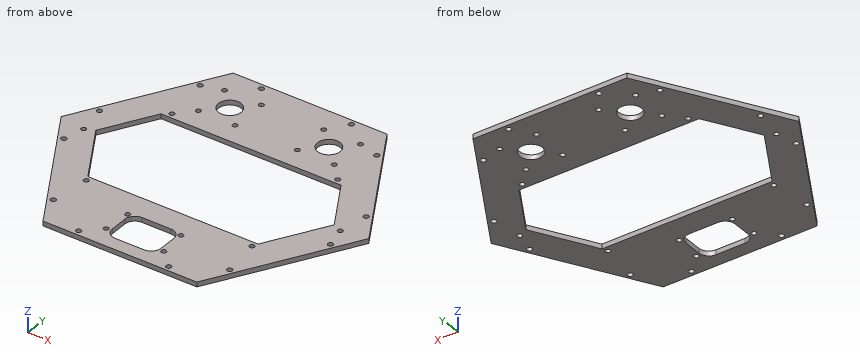
from build123d import *

# Parameters (mm, degrees)
FLANGE_BASE1_DEPTH          = 3.175
ESBO_O6_R                   = 1.65
CORTE_EXTRUS_O1_DEPTH       = 10
ESBO_O7_R                   = 1.75
CORTE_EXTRUS_O2_DEPTH       = 10
ESBO_O8_R                   = 7.554969153
ESBO_O8_R_2                 = 1.65
CORTE_EXTRUS_O3_DEPTH       = 10
PADR_OCIRCULAR1_COUNT       = 4
PADR_OCIRCULAR2_COUNT       = 6
ESPELHAR1_COPY_1_SKETCH_R   = 7.554969153
ESPELHAR1_COPY_1_SKETCH_R_2 = 1.65
ESPELHAR1_COPY_1_DEPTH      = 10
ESPELHAR1_COPY_2_SKETCH_R   = 7.554969153
ESPELHAR1_COPY_2_SKETCH_R_2 = 1.65
ESPELHAR1_COPY_2_DEPTH      = 10
ESPELHAR1_COPY_3_SKETCH_R   = 7.554969153
ESPELHAR1_COPY_3_SKETCH_R_2 = 1.65
ESPELHAR1_COPY_3_DEPTH      = 10
ESBO_O9_R                   = 1.65
CORTE_EXTRUS_O4_DEPTH       = 10


# Sheet-metal steps are written as plain solids
with BuildPart() as part:
    # Esboço1 → Flange-base1 (new body)
    with BuildSketch(Plane.XY):
        Polygon((51.251383396, 88.77), (102.502766792, 0), (51.251383396, -88.77), (-51.251383396, -88.77), (-102.502766792, 0), (-51.251383396, 88.77), align=None)
        Polygon((60, 33.616951546), (-60, 33.616951546), (-79.408756024, 0), (-56.734237399, -39.273418297), (56.734237399, -39.273418297), (79.408756024, 0), align=None, mode=Mode.SUBTRACT)
    extrude(amount=-FLANGE_BASE1_DEPTH)

    # Esboço6 → Corte-extrusão1 (cut)
    with BuildSketch(Plane.XY):
        with BuildLine():
            Line((9.692826752, -79.77), (-9.607173248, -79.77))
            ThreePointArc((-9.607173248, -79.77), (-14.274078004, -77.836904756), (-16.207173248, -73.17))
            Line((-16.207173248, -73.17), (-16.207173248, -61.37))
            ThreePointArc((-16.207173248, -61.37), (-14.274078004, -56.703095244), (-9.607173248, -54.77))
            Line((-9.607173248, -54.77), (9.692826752, -54.77))
            ThreePointArc((9.692826752, -54.77), (14.359731508, -56.703095244), (16.292826752, -61.37))
            Line((16.292826752, -61.37), (16.292826752, -73.17))
            ThreePointArc((16.292826752, -73.17), (14.359731508, -77.836904756), (9.692826752, -79.77))
        make_face()
        with Locations((-17.7, -56.67)):
            Circle(ESBO_O6_R)
        with Locations((17.7, -56.67)):
            Circle(ESBO_O6_R)
        with Locations((19.2, -74.77)):
            Circle(ESBO_O6_R)
        with Locations((-19.2, -74.77)):
            Circle(ESBO_O6_R)
    extrude(amount=-CORTE_EXTRUS_O1_DEPTH, mode=Mode.SUBTRACT)

    # Esboço7 → Corte-extrusão2 (cut)
    with BuildSketch(Plane.XY):
        with Locations((-30, -85.27)):
            Circle(ESBO_O7_R)
        with Locations((30, -85.27)):
            Circle(ESBO_O7_R)
    corte_extrus_o2 = extrude(amount=-CORTE_EXTRUS_O2_DEPTH, mode=Mode.SUBTRACT)

    # Esboço8 → Corte-extrusão3 (cut)
    with BuildSketch(Plane.XY):
        with Locations((-33, 60.0982)):
            Circle(ESBO_O8_R)
        with Locations((-20.75, 47.8482)):
            Circle(ESBO_O8_R_2)
    corte_extrus_o3 = extrude(amount=-CORTE_EXTRUS_O3_DEPTH, mode=Mode.SUBTRACT)

    # PadrãoCircular1: Corte-extrusão3 ×4 about axis
    padr_ocircular1_axis = Axis((-33, 60.0982, 0), (0, 0, 1))
    for i in range(1, PADR_OCIRCULAR1_COUNT):
        add(corte_extrus_o3.rotate(padr_ocircular1_axis, i * 360 / PADR_OCIRCULAR1_COUNT), mode=Mode.SUBTRACT)

    # PadrãoCircular2: Corte-extrusão2 ×6 about axis
    padr_ocircular2_axis = Axis((0, 0, 0), (0, 0, 1))
    for i in range(1, PADR_OCIRCULAR2_COUNT):
        add(corte_extrus_o2.rotate(padr_ocircular2_axis, i * 360 / PADR_OCIRCULAR2_COUNT), mode=Mode.SUBTRACT)

    # Espelhar1: Corte-extrusão3 across plane
    add(corte_extrus_o3.mirror(Plane(origin=(0, 0, 0), x_dir=(0, 0, 1), z_dir=(1, 0, 0))), mode=Mode.SUBTRACT)

    # Espelhar1 copy 1 sketch → Espelhar1 copy 1 (cut)
    with BuildSketch(Plane(origin=(-27.0982, 93.0982, 0), x_dir=(0, 1, 0), z_dir=(0, 0, 1))):
        with Locations((-33, -60.0982)):
            Circle(ESPELHAR1_COPY_1_SKETCH_R)
        with Locations((-20.75, -47.8482)):
            Circle(ESPELHAR1_COPY_1_SKETCH_R_2)
    extrude(amount=-ESPELHAR1_COPY_1_DEPTH, mode=Mode.SUBTRACT)

    # Espelhar1 copy 2 sketch → Espelhar1 copy 2 (cut)
    with BuildSketch(Plane(origin=(66, 120.1964, 0), x_dir=(1, 0, 0), z_dir=(0, 0, 1))):
        with Locations((-33, -60.0982)):
            Circle(ESPELHAR1_COPY_2_SKETCH_R)
        with Locations((-20.75, -47.8482)):
            Circle(ESPELHAR1_COPY_2_SKETCH_R_2)
    extrude(amount=-ESPELHAR1_COPY_2_DEPTH, mode=Mode.SUBTRACT)

    # Espelhar1 copy 3 sketch → Espelhar1 copy 3 (cut)
    with BuildSketch(Plane(origin=(93.0982, 27.0982, 0), x_dir=(0, -1, 0), z_dir=(0, 0, 1))):
        with Locations((-33, -60.0982)):
            Circle(ESPELHAR1_COPY_3_SKETCH_R)
        with Locations((-20.75, -47.8482)):
            Circle(ESPELHAR1_COPY_3_SKETCH_R_2)
    extrude(amount=-ESPELHAR1_COPY_3_DEPTH, mode=Mode.SUBTRACT)

    # Esboço9 → Corte-extrusão4 (cut)
    with BuildSketch(Plane.XY):
        with Locations((-55.257737945, 37.171766625)):
            Circle(ESBO_O9_R)
        with Locations((-85.480762114, -2.828233375)):
            Circle(ESBO_O9_R)
        with Locations((85.480762114, -2.828233375)):
            Circle(ESBO_O9_R)
        with Locations((55.257737945, 37.171766625)):
            Circle(ESBO_O9_R)
        with Locations((55.257737945, -42.828233375)):
            Circle(ESBO_O9_R)
        with Locations((-55.257737945, -42.828233375)):
            Circle(ESBO_O9_R)
    extrude(amount=-CORTE_EXTRUS_O4_DEPTH, mode=Mode.SUBTRACT)


solid = part.part
Geometry check sheet. Reference: the model listing, model coordinates, mm. Give positions to 0.01 mm unless a question says otherwise; leave off trailing zeros. Order: outer loops, then holes, each group sorted by start corner. A loop starts at its lowest first (then second) coordinate and runs counter-clockwise, first axis right, second up. Notation, with made-up numbers: M 48,68 L 90,68 A29 ccw 90,98 Z; hole C 89,86.25 d4. An arc over 180 degrees is marked long. Use a Markdown table: item, result.
Item 1: Depth check by flat-ended pin: P1, Ø13.5, axis at x = -33, y = 60.1, coming from the -Z side. Enter the tip coordinate at first touch or a pass-through.
Answers follow:
| item | result |
|---|---|
| P1 | passes through |
Item 2: Section check A-A (y = 55). Record the cut outline in (x, z) (1 decimal), and give its area (3 significant figures).
Answers follow:
| item | result |
|---|---|
| outline | M -70.7,-3.2 L -38.6,-3.2 L -38.6,0 L -70.7,0 Z; M -27.4,-3.2 L 27.4,-3.2 L 27.4,0 L -27.4,0 Z; M 38.6,-3.2 L 70.7,-3.2 L 70.7,0 L 38.6,0 Z |
| area | 378 mm2 |
Item 3: Section check D-D (z = -2.05). State how many separate pieces and enclosed holes the cut face has, and give its area (3 significant figures).
Answers follow:
| item | result |
|---|---|
| separate pieces | 1 |
| enclosed holes | 34 |
| area | 15,900 mm2 |
Item 4: Section check C-C (y = -21). Record the cut outline in (x, z) (3 decimals).
Answers follow:
| item | result |
|---|---|
| outline | M -90.378,-3.175 L -67.284,-3.175 L -67.284,0 L -90.378,0 Z; M 67.284,-3.175 L 90.378,-3.175 L 90.378,0 L 67.284,0 Z |
Item 5: Section check B-B (x = 67.5). Record the cut outline in (y, z) (3 decimals).
Answers follow:
| item | result |
|---|---|
| outline | M -60.627,-3.175 L -20.627,-3.175 L -20.627,0 L -60.627,0 Z; M 20.627,-3.175 L 60.627,-3.175 L 60.627,0 L 20.627,0 Z |
Item 6: Material ranges on line 1 along Y through (x, z) = (4, -2.3); line 2 along X through (y, z) = (61.5, -0.75); line 3 along Y through (x, z) = (59, -2.4), recorded low to high.
Answers follow:
| item | result |
|---|---|
| line 1 | y = -88.77 to -79.77, -54.77 to -39.27, 33.62 to 88.77 |
| line 2 | x = -67 to -40.42, -25.58 to 25.58, 40.42 to 67 |
| line 3 | y = -75.35 to -70.36, -66.87 to -35.35, 33.62 to 66.87, 70.36 to 75.35 |
